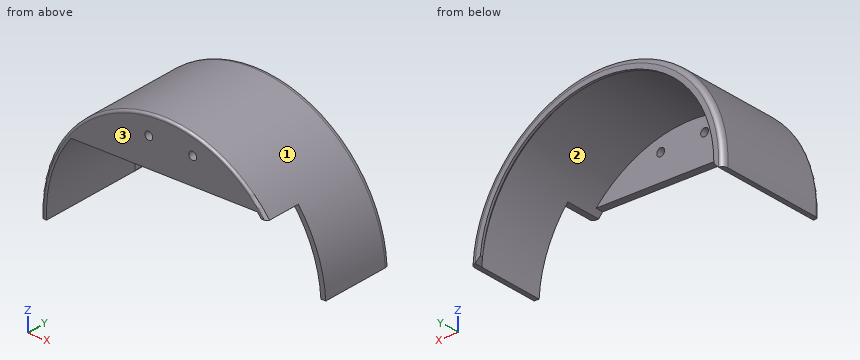
```python
from build123d import *

# Parameters (mm, degrees)
BOX338_W                = 59
BOX338_H                = 20
BOX338_DEPTH            = 32
BOX338_PLACEMENT_ANGLE  = 3
CYLINDER483_R           = 1.6
CYLINDER483_DEPTH       = 9
CYLINDER481_R           = 1.6
CYLINDER481_DEPTH       = 9
BOX337_W                = 128
BOX337_H                = 3
BOX337_DEPTH            = 35
BOX337_PLACEMENT_ANGLE  = 3
CYLINDER489_W           = 52
CYLINDER489_H           = 3
CYLINDER489_ANGLE       = 180
CYLINDER489_ROLL_ANGLE  = 90
CYLINDER489_PITCH_ANGLE = -3
CYLINDER491_W           = 48
CYLINDER491_H           = 2
CYLINDER491_ANGLE       = 180
CYLINDER488_W           = 50
CYLINDER488_H           = 42
CYLINDER488_ANGLE       = 180
CYLINDER490_W           = 52
CYLINDER490_H           = 43
CYLINDER490_ANGLE       = 180
CUT342_PLACEMENT_ANGLE  = 3
FILLET124_R             = 2
FILLET125_R             = 1
CHAMFER049_SIZE         = 1.99
CHAMFER052_SIZE         = 1.99


with BuildPart() as cube409:
    # Box338 → Box338 (new body)
    with BuildSketch(Plane.XY):
        with Locations((29.5, 10)):
            Rectangle(BOX338_W, BOX338_H)
    extrude(amount=BOX338_DEPTH)


with BuildPart() as cube409_1:
    # Box338 placement: moved
    add(cube409.part.moved(Location((473, -33, -34))).rotate(Axis((473, -33, -34), (0, -1, 0)), BOX338_PLACEMENT_ANGLE))


with BuildPart() as cylinder584:
    # Cylinder483 → Cylinder483 (new body)
    with BuildSketch(Plane(origin=(441, -17, 10), x_dir=(1, 0, 0), z_dir=(0, -1, 0))):
        Circle(CYLINDER483_R)
    extrude(amount=CYLINDER483_DEPTH)


with BuildPart() as fusion433:
    # Cylinder481 → Cylinder481 (new body)
    with BuildSketch(Plane(origin=(459, -17, 10), x_dir=(1, 0, 0), z_dir=(0, -1, 0))):
        Circle(CYLINDER481_R)
    extrude(amount=CYLINDER481_DEPTH)

    # Fusion433: union Cylinder584
    add(cylinder584.part)


with BuildPart() as cube408:
    # Box337 → Box337 (new body)
    with BuildSketch(Plane.XY):
        with Locations((64, 1.5)):
            Rectangle(BOX337_W, BOX337_H)
    extrude(amount=BOX337_DEPTH)


with BuildPart() as cube408_1:
    # Box337 placement: moved
    add(cube408.part.moved(Location((382, -9, -40.8))).rotate(Axis((382, -9, -40.8), (0, -1, 0)), BOX337_PLACEMENT_ANGLE))


with BuildPart() as cut343:
    # Cylinder489 → Cylinder489 (revolve)
    with BuildSketch(Plane.XZ):
        with Locations((26, 1.5)):
            Rectangle(CYLINDER489_W, CYLINDER489_H)
    revolve(axis=Axis((0, 0, 0), (0, 0, 1)), revolution_arc=CYLINDER489_ANGLE)


with BuildPart() as cut343_1:
    # Cylinder489 roll: moved
    add(cut343.part.rotate(Axis((0, 0, 0), (1, 0, 0)), CYLINDER489_ROLL_ANGLE))


with BuildPart() as cut343_2:
    # Cylinder489 pitch: moved
    add(cut343_1.part.rotate(Axis((0, 0, 0), (0, 1, 0)), CYLINDER489_PITCH_ANGLE))


with BuildPart() as cut343_3:
    # Cylinder489 placement: moved
    add(cut343_2.part.moved(Location((448.581401, -6, -35.39126))))

    # Cut343: cut Cube408
    add(cube408_1.part, mode=Mode.SUBTRACT)


with BuildPart() as cut343_4:
    # Cut343 placement: moved
    add(cut343_3.part.moved(Location((105.48, -13, 6.5))))


with BuildPart() as cylinder588:
    # Cylinder491 → Cylinder491 (revolve)
    with BuildSketch(Plane(origin=(554, -60, -28), x_dir=(1, 0, 0), z_dir=(0, 0, -1))):
        with Locations((24, 1)):
            Rectangle(CYLINDER491_W, CYLINDER491_H)
    revolve(axis=Axis((554, -60, -28), (0, -1, 0)), revolution_arc=CYLINDER491_ANGLE)


with BuildPart() as fusion438:
    # Cylinder488 → Cylinder488 (revolve)
    with BuildSketch(Plane(origin=(554, -19, -28), x_dir=(1, 0, 0), z_dir=(0, 0, -1))):
        with Locations((25, 21)):
            Rectangle(CYLINDER488_W, CYLINDER488_H)
    revolve(axis=Axis((554, -19, -28), (0, -1, 0)), revolution_arc=CYLINDER488_ANGLE)

    # Fusion438: union Cylinder588
    add(cylinder588.part)


with BuildPart() as fender_front_left:
    # Cylinder490 → Cylinder490 (revolve)
    with BuildSketch(Plane(origin=(554, -19, -28), x_dir=(1, 0, 0), z_dir=(0, 0, -1))):
        with Locations((26, 21.5)):
            Rectangle(CYLINDER490_W, CYLINDER490_H)
    revolve(axis=Axis((554, -19, -28), (0, -1, 0)), revolution_arc=CYLINDER490_ANGLE)

    # Cut342: cut Fusion438
    add(fusion438.part, mode=Mode.SUBTRACT)


with BuildPart() as fender_front_left_1:
    # Cut342 placement: moved
    add(fender_front_left.part.moved(Location((-0.706169, 0, -29.032493))).rotate(Axis((-0.706169, 0, -29.032493), (0, -1, 0)), CUT342_PLACEMENT_ANGLE))

    # Fusion437: union Cut343
    add(cut343_4.part)


with BuildPart() as fender_front_left_2:
    # Fusion437 placement: moved
    add(fender_front_left_1.part.moved(Location((-105, 0, -5.5))))

    # Cut345: cut Fusion433
    add(fusion433.part, mode=Mode.SUBTRACT)

    # Cut347: cut Cube409
    add(cube409_1.part, mode=Mode.SUBTRACT)

    # Fillet124
    fillet124_edges = [fender_front_left_2.edges().sort_by_distance(p)[0] for p in [
        (446.27853, -62, 18.428736),
    ]]
    fillet(fillet124_edges, radius=FILLET124_R)

    # Fillet125
    fillet125_edges = [fender_front_left_2.edges().sort_by_distance(p)[0] for p in [
        (430.549251, -19, 15.116559),
    ]]
    fillet(fillet125_edges, radius=FILLET125_R)

    # Chamfer049
    chamfer049_edges = [fender_front_left_2.edges().sort_by_distance(p)[0] for p in [
        (446.383202, -61, 16.431477),
    ]]
    chamfer(chamfer049_edges, length=CHAMFER049_SIZE)

    # Chamfer052
    chamfer052_edges = [fender_front_left_2.edges().sort_by_distance(p)[0] for p in [
        (401.065782, -61.5, -36.012126),
        (496.934218, -61.5, -30.987874),
    ]]
    chamfer(chamfer052_edges, length=CHAMFER052_SIZE)


with BuildPart() as fender_front_right:
    # Part__Mirroring011: instance of fender-front-left_
    add(fender_front_left_2.part.mirror(Plane(origin=(0, 0, 0), x_dir=(1, 0, 0), z_dir=(0, 1, 0))))


with BuildPart() as fender_front_right_1:
    # Part__Mirroring011 placement: moved
    add(fender_front_right.part.moved(Location((0, 62, 0))))


solid = fender_front_right_1.part
```
Geometry: final body of the model. Coordinates: model frame, mm. Face numbers are marked on the shaded views. Round coordinates to 2 decimals unless told otherwise and drop trailing zeros. Write each loop counter-clockwise with the first axis right and the second up, starting at its lowest first coordinate (ties: lowest second). Pieces come first, ordered by that corner, then holes.
Item 1: Material intervals for L1, parallel to X at y = 81.75, z = 10; L2, parallel to X at y = 81.85, z = 10; L3, parallel to X at y = 117.5, z = -14.5, sorted ascending.
Item 2: Pin query (flat end, axial travel): P1, Ø2, axis at y = 107.5, z = -5, coming from the +X side; P2, Ø10, axis at y = 91.5, z = 7, coming from the -X side; P3, Ø2.5, axis at x = 459, z = 10, coming from the +Y side; P4, Ø5, axis at x = 441, z = 10, coming from the +Y side. Return the tip coordinate at first contact, or that it passes through.
Item 3: Mould query, pull axis X, two halves, no side actions, for the marked faces 1, 2 and 3. Classes: +X half, -X half, draft (parallel to the pull), parting line (faces both ways), or undercut.
Item 4: Section query A-A (y = 86). Return loops of the section in (x, z).
Completed:
1. L1: x = 420.57 to 439.4, 442.6 to 457.4, 460.6 to 477.43
1. L2: x = 420.53 to 439.4, 442.6 to 457.4, 460.6 to 477.47
1. L3: x = 400.6 to 402.75, 495.25 to 497.4
2. P1: stops at x = 493.13
2. P2: stops at x = 411
2. P3: passes through
2. P4: stops at y = 84
3. face 1: parting line
3. face 2: undercut
3. face 3: draft
4. outline: (397.07, -36.22) - (399.07, -36.12) arc R50 cw to (487.18, -1.21) - (489.66, -1.08) arc R52 ccw to start
